Geometry check sheet. Reference: drawing and pictorial views, mm from the part's lowest x, y, z. A direction names the side the tool comes from. Round coordinates to 2 decimals unless told otherwise and drop trailing zeros. Write each loop counter-clockwise with the first axis right and the second up, starting at its lowest first coordinate (ties: lowest second). Pieces come first, ordered by that corner, then holes. Notation, with made-up numbers: (52.25, -6.75) -> (104.25, -6.75) arc R24 ccw to (104.25, 11.25) -> close; hole circle Ø8 at (-5.5, 67). An arc over 180 degrees is marked (long way). Write item = value, one per line.
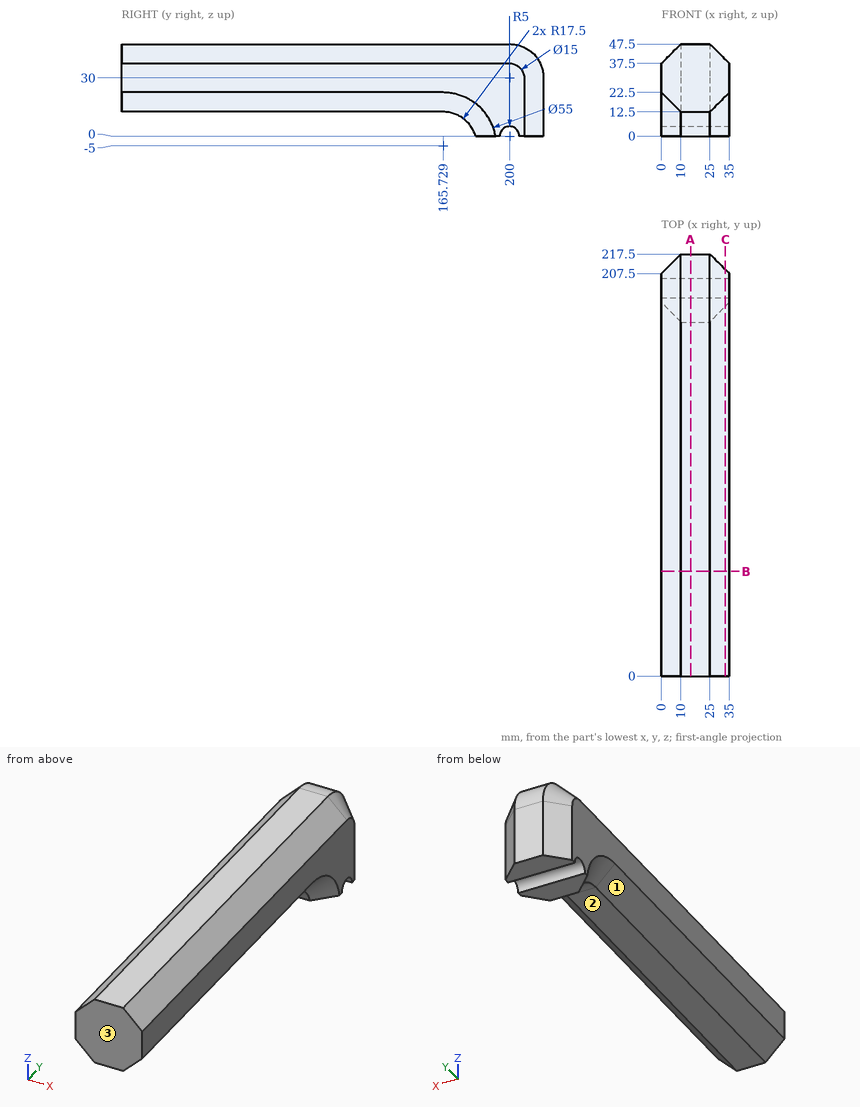
(1) Sectioned sample at C-C on x = 33. Enter the section's corners in (y, z) (1 decimal).
Worked answers:
outline = (0, 20.5) -> (165.7, 20.5) arc R25.5 cw to (190.7, 0) -> (195, 0) arc R5 cw to (205, 0) -> (209.5, 0) -> (209.5, 30) arc R9.5 ccw to (200, 39.5) -> (0, 39.5) -> close
(2) Access from +Z, -Z, +X, -X, +Y, -Y to the whole of each face (thin tool, end or side, straight path). Record for the marked faces 1, 2 and 3.
Worked answers:
face_1 = -Z, -X, -Y
face_2 = -Z, +X, -X, -Y
face_3 = +Z, -Z, +X, -X, -Y
(3) Material ranges on L1, parallel to Z at x = 23, y = 98; L2, parallel to Y at x = 24.5, z = 3.5 (1 decimal); L3, parallel to Y at x = 7, z = 6, recorded low to high. Write a range as [from, to].
Worked answers:
L1 = [12.5, 47.5]
L2 = [181, 196.4], [203.6, 217.5]
L3 = [183.03, 214.5]
(4) Go/stop test with a flat-tipped pin: P1, Ø10, axis at x = 15.5, y = 71, coming from the -Z side. Record where the tip stops, or that it passes through.
Worked answers:
P1 = 12.5
(5) Sectioned sample at B-B on y = 54. Enter the section's corners in (x, z).
Worked answers:
outline = (0, 22.5) -> (10, 12.5) -> (25, 12.5) -> (35, 22.5) -> (35, 37.5) -> (25, 47.5) -> (10, 47.5) -> (0, 37.5) -> close
(6) Sectioned sample at A-A on x = 15. Enter the section's corners in (y, z).
Worked answers:
outline = (0, 12.5) -> (165.73, 12.5) arc R17.5 cw to (182.5, 0) -> (195, 0) arc R5 cw to (205, 0) -> (217.5, 0) -> (217.5, 30) arc R17.5 ccw to (200, 47.5) -> (0, 47.5) -> close
